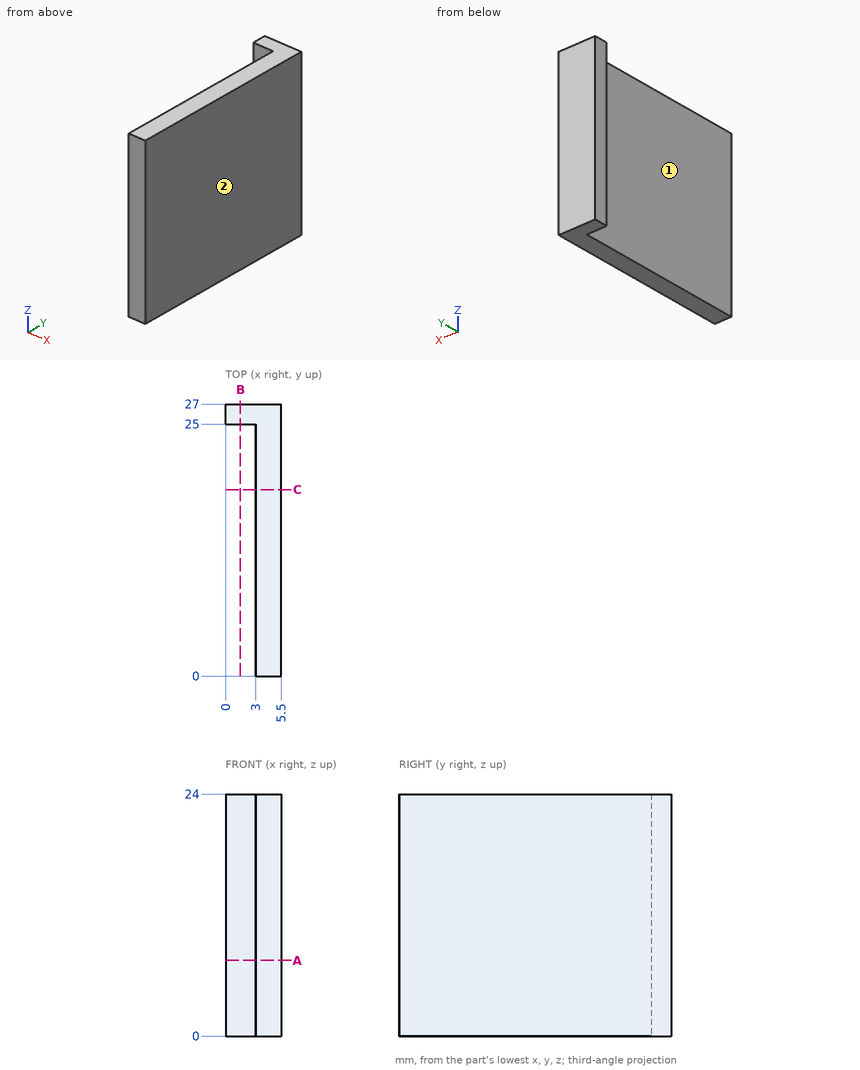
Part print with two shaded views. Sizes in mm from the minimum x, y, z corner. A direction names the side the tool comes from. Give positions to 0.01 mm unless a question says otherwise; leave off trailing zeros. Order: outer loops, then holes, each group sorted by start corner. A loop starts at its lowest first (then second) coordinate and runs counter-clockwise, first axis right, second up. Notation, with made-up numbers: M 67,19.25 L 96,19.25 A25 cw 96,48.25 Z; hole C 13.5,3 d9. An arc over 180 degrees is marked long. Write item = value, one per line.
Q1. Flat gauge pins, fed straight in: pin 1 (12 mm diameter, centred on y = 3.5, z = 9.5, fed in from -X); pin 2 (2.5 mm diameter, centred on x = 2, z = 16.5, fed in from -Y). Where does each tip first touch, or does it go through?
Derived:
pin_1 = 3
pin_2 = 0
Q2. Drill centre lines: line 1 (X direction, y = 16.5, z = 18); line 2 (Y direction, x = 1.4, z = 23.25). Where is each one in solid material? Low to high. Write a range as [from, to].
Derived:
line_1 = [3, 5.5]
line_2 = [25, 27]
Q3. Cut at A-A, the plane z = 7.5. List the corners of the cut face in (x, y), then the cut area to 3 significant figures.
Derived:
outline = M 0,25 L 3,25 L 3,0 L 5.5,0 L 5.5,27 L 0,27 Z
area = 73.5 mm2
Q4. Tool access for the marked faces 1 and 2: list every direction of +Z, -Z, +X, -X, +Y, -Y with a clear straight run to the whole face (end or side of a thin tool).
Derived:
face_1 = +Z, -Z, -X, -Y
face_2 = +Z, -Z, +X, +Y, -Y
Q5. Cut at B-B, the plane x = 1.45. List the corners of the cut face in (y, z).
Derived:
outline = M 25,0 L 27,0 L 27,24 L 25,24 Z
Q6. Cut at C-C, the plane y = 18.5. List the corners of the cut face in (x, z), then the cut area to 3 significant figures.
Derived:
outline = M 3,0 L 5.5,0 L 5.5,24 L 3,24 Z
area = 60.0 mm2
